```python
from build123d import *

# Parameters (mm, degrees)
BOSS_EXTRUDE1_DEPTH = 260
SKETCH2_R           = 3
CUT_EXTRUDE1_DEPTH  = 4.5
SKETCH3_R           = 1.75
CUT_EXTRUDE2_DEPTH  = 261.192236625


with BuildPart() as part:
    # Sketch1 → Boss-Extrude1 (new body)
    with BuildSketch(Plane.XY):
        with BuildLine():
            Line((-5.6, 4), (5.6, 4))
            ThreePointArc((5.6, 4), (5.882842712, 3.882842712), (6, 3.6))
            Line((6, 3.6), (6, 2.8))
            Line((6, 2.8), (5.2, 2))
            Line((5.2, 2), (4.4, 2))
            Line((4.4, 2), (4.4, 1))
            Line((4.4, 1), (5.2, 1))
            Line((5.2, 1), (6, 0.2))
            Line((6, 0.2), (6, -3.6))
            ThreePointArc((6, -3.6), (5.882842712, -3.882842712), (5.6, -4))
            Line((5.6, -4), (-5.6, -4))
            ThreePointArc((-5.6, -4), (-5.882842712, -3.882842712), (-6, -3.6))
            Line((-6, -3.6), (-6, 0.2))
            Line((-6, 0.2), (-5.2, 1))
            Line((-5.2, 1), (-4.4, 1))
            Line((-4.4, 1), (-4.4, 2))
            Line((-4.4, 2), (-5.2, 2))
            Line((-5.2, 2), (-6, 2.8))
            Line((-6, 2.8), (-6, 3.6))
            ThreePointArc((-6, 3.6), (-5.882842712, 3.882842712), (-5.6, 4))
        make_face()
    extrude(amount=BOSS_EXTRUDE1_DEPTH)

    # Sketch2 → Cut-Extrude1 (cut)
    with BuildSketch(Plane(origin=(0, 4, 0), x_dir=(1, 0, 0), z_dir=(0, 1, 0))):
        with Locations(Location((0, -242.5, 0), (0, 0, 270))):
            Circle(SKETCH2_R)
        with Locations(Location((0, -217.5, 0), (0, 0, 270))):
            Circle(SKETCH2_R)
        with Locations(Location((0, -192.5, 0), (0, 0, 270))):
            Circle(SKETCH2_R)
        with Locations(Location((0, -167.5, 0), (0, 0, 270))):
            Circle(SKETCH2_R)
        with Locations(Location((0, -142.5, 0), (0, 0, 270))):
            Circle(SKETCH2_R)
        with Locations(Location((0, -117.5, 0), (0, 0, 270))):
            Circle(SKETCH2_R)
        with Locations(Location((0, -92.5, 0), (0, 0, 270))):
            Circle(SKETCH2_R)
        with Locations(Location((0, -67.5, 0), (0, 0, 270))):
            Circle(SKETCH2_R)
        with Locations(Location((0, -42.5, 0), (0, 0, 270))):
            Circle(SKETCH2_R)
        with Locations(Location((0, -17.5, 0), (0, 0, 270))):
            Circle(SKETCH2_R)
        with Locations((0, 7.5)):
            Circle(SKETCH2_R)
        with Locations((0, 32.5)):
            Circle(SKETCH2_R)
        with Locations((0, 57.5)):
            Circle(SKETCH2_R)
        with Locations((0, 82.5)):
            Circle(SKETCH2_R)
        with Locations((0, 107.5)):
            Circle(SKETCH2_R)
        with Locations((0, 132.5)):
            Circle(SKETCH2_R)
        with Locations((0, 157.5)):
            Circle(SKETCH2_R)
        with Locations((0, 182.5)):
            Circle(SKETCH2_R)
    extrude(amount=-CUT_EXTRUDE1_DEPTH, mode=Mode.SUBTRACT)

    # Sketch3 → Cut-Extrude2 (cut, through all)
    with BuildSketch(Plane(origin=(0, 4, 0), x_dir=(1, 0, 0), z_dir=(0, 1, 0))):
        with Locations(Location((0, -242.5, 0), (0, 0, 270))):
            Circle(SKETCH3_R)
        with Locations(Location((0, -217.5, 0), (0, 0, 270))):
            Circle(SKETCH3_R)
        with Locations(Location((0, -192.5, 0), (0, 0, 270))):
            Circle(SKETCH3_R)
        with Locations(Location((0, -167.5, 0), (0, 0, 270))):
            Circle(SKETCH3_R)
        with Locations(Location((0, -142.5, 0), (0, 0, 270))):
            Circle(SKETCH3_R)
        with Locations(Location((0, -117.5, 0), (0, 0, 270))):
            Circle(SKETCH3_R)
        with Locations(Location((0, -92.5, 0), (0, 0, 270))):
            Circle(SKETCH3_R)
        with Locations(Location((0, -67.5, 0), (0, 0, 270))):
            Circle(SKETCH3_R)
        with Locations(Location((0, -42.5, 0), (0, 0, 270))):
            Circle(SKETCH3_R)
        with Locations(Location((0, -17.5, 0), (0, 0, 270))):
            Circle(SKETCH3_R)
        with Locations((0, 7.5)):
            Circle(SKETCH3_R)
        with Locations((0, 32.5)):
            Circle(SKETCH3_R)
        with Locations((0, 57.5)):
            Circle(SKETCH3_R)
        with Locations((0, 82.5)):
            Circle(SKETCH3_R)
        with Locations((0, 107.5)):
            Circle(SKETCH3_R)
    extrude(amount=-CUT_EXTRUDE2_DEPTH, mode=Mode.SUBTRACT)


solid = part.part
```
CAD build for the part. Positions are in the model's coordinates, mm. A direction names the side the tool comes from. Give positions to 0.01 mm unless a question says otherwise; leave off trailing zeros. Write each loop counter-clockwise with the first axis right and the second up, starting at its lowest first coordinate (ties: lowest second). Pieces come first, ordered by that corner, then holes. Notation, with made-up numbers: (56.5, -2.5) -> (83.5, -2.5) arc R17 cw to (83.5, 14.5) -> close; hole circle Ø11 at (-37, 63). An arc over 180 degrees is marked (long way). Write each question's results on one line, items separated by ' | '.
1. Cut at A-A, the plane z = 178.5. Write the cut outline in (x, y).
Geometry check:
outline: (-6, -3.6) arc R0.4 ccw to (-5.6, -4) -> (5.6, -4) arc R0.4 ccw to (6, -3.6) -> (6, 0.2) -> (5.2, 1) -> (4.4, 1) -> (4.4, 2) -> (5.2, 2) -> (6, 2.8) -> (6, 3.6) arc R0.4 ccw to (5.6, 4) -> (-5.6, 4) arc R0.4 ccw to (-6, 3.6) -> (-6, 2.8) -> (-5.2, 2) -> (-4.4, 2) -> (-4.4, 1) -> (-5.2, 1) -> (-6, 0.2) -> close
2. Cut at B-B, the plane y = -2. Give the number of separate pieces and of enclosed holes in the cut face, then the cut area to 3 significant figures.
Geometry check:
separate pieces: 1 | enclosed holes: 10 | area: 3,020 mm²
3. Wall check: probe 1 along X at (y, z) = (1.8, 117.5); probe 2 along Y at (x, z) = (-5, 93.5); probe 3 along X at (y, z) = (-1.9, 217.5). Give the ranges that are in metal, low to high. Write a range as [from, to].
Geometry check:
probe 1: [-4.4, -3], [3, 4.4] | probe 2: [-4, 1], [2, 4] | probe 3: [-6, -1.75], [1.75, 6]
4. Two-plate mould, pull along X, no slides. Class faces 1 (the flat face through (0, 0, 0)), 2 (the cylindrical face through (-1.8, 1.8, 65.1)), 3 (the cylindrical face through (0.9, 1.78, 145.36)): pulls with the +X half, pulls with the -X half, needs draft (parallel to the pull), parting line crosses it, or undercut.
Geometry check:
face 1: needs draft | face 2: undercut | face 3: undercut
5. Drop flat-ended pins along their axis: P1, Ø4.5, axis at x = 0, z = 217.5, coming from the +Y side; P2, Ø3, axis at x = 0, z = 117.5, coming from the +Y side; P3, Ø0.8, axis at y = 1.5, z = 157.5, coming from the -X side. Give the stop position or say it passes through.
Geometry check:
P1: y = -0.5 | P2: through | P3: x = -4.4
6. Which spindle directions (+Z, -Z, +X, -X, +Y, -Y) get a long thin tool onto all of the face, cutting with end or side? Do faces 4 (the flat face through (-2, -0.5, 192)), 5 (the flat face through (0, -4, 128)). Say none if no direction does.
Geometry check:
face 4: +Y | face 5: +Z, -Z, +X, -X, -Y
